Could you check a few things on this model? Use its own coordinates, in mm. Face numbers are marked on the shaded views. A direction names the side the tool comes from. Give positions to 0.01 mm unless a question says otherwise; leave off trailing zeros. Write each loop counter-clockwise with the first axis right and the second up, starting at its lowest first coordinate (ties: lowest second). Pieces come first, ordered by that corner, then holes. Notation, with made-up numbers: M 88,73 L 138,73 A24 ccw 138,98 Z; hole C 38.25,48 d2. An arc over 180 degrees is marked long. One line per item, written item: value.
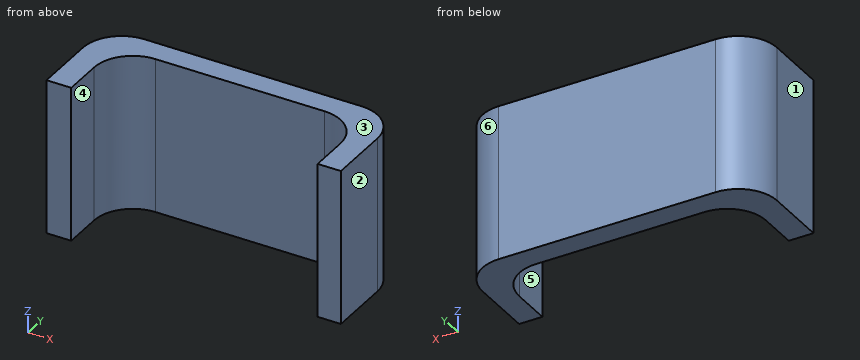
```python
from build123d import *

# Parameters (mm, degrees)
EXTRUDE_1_DEPTH = 40


with BuildPart() as part:
    # 草图1 → 凸台-拉伸1 (new body)
    with BuildSketch(Plane.XY):
        with BuildLine():
            Line((-37.999999813, 14.005326892), (-37.999999813, 20.009487218))
            Line((-37.999999813, 20.009487218), (-37.999999813, 30))
            ThreePointArc((-37.999999813, 30), (-35.071067625, 37.071067812), (-27.999999813, 40))
            Line((-27.999999813, 40), (28, 40))
            ThreePointArc((28, 40), (35.071067812, 37.071067812), (38, 30))
            Line((38, 30), (38, 20))
            Line((38, 20), (38, 14))
            Line((38, 14), (32, 14))
            Line((32, 14), (32, 24))
            ThreePointArc((32, 24), (29.071067812, 31.071067812), (22, 34))
            Line((22, 34), (-21.616055892, 34))
            ThreePointArc((-21.616055892, 34), (-28.687123704, 31.071067812), (-31.616055892, 24))
            Line((-31.616055892, 24), (-31.616055892, 14.005326892))
            Line((-31.616055892, 14.005326892), (-37.999999813, 14.005326892))
        make_face()
    extrude(amount=EXTRUDE_1_DEPTH)


solid = part.part
```
1) I'm going to push flat-ended pins straight in: pin 1 (10 mm diameter, centred on y = 33.5, z = 13.5, fed in from +X); pin 2 (8 mm diameter, centred on x = -10.5, z = 4, fed in from -Y); pin 3 (3 mm diameter, centred on x = -33.5, z = 26.5, fed in from -Y). Where does each tip first touch, or does it pass through?
Outcome:
pin 1: stops at x = 38
pin 2: stops at y = 34
pin 3: stops at y = 14.01
2) If we section it at D-D, the plane y = 26.5: Write out the boundary of the cut face in (x, z).
Outcome:
outline: M -38,0 L -31.3,0 L -31.3,40 L -38,40 Z; M 31.68,0 L 38,0 L 38,40 L 31.68,40 Z
3) We'd pull the mould along X, two halves only. Please class the marked faces 1, 2, 3 and 4: pulls with the +X half, pulls with the -X half, needs draft (parallel to the pull), parting line crosses it, or undercut.
Outcome:
face 1: pulls with the -X half
face 2: pulls with the +X half
face 3: needs draft
face 4: undercut
4) If we section it at A-A, the plane y = 21.25: Write out the boundary of the cut face in (x, z).
Outcome:
outline: M -38,0 L -31.62,0 L -31.62,40 L -38,40 Z; M 32,0 L 38,0 L 38,40 L 32,40 Z
5) If we section it at C-C, the plane x = 12: Write out the boundary of the cut face in (y, z), then the cut area to 3 significant figures.
Outcome:
outline: M 34,0 L 40,0 L 40,40 L 34,40 Z
area: 240 mm^2
6) On a 3-axis mill with a long thin cutter (end or side, diameter ignored), from which of +Z, -Z, +X, -X, +Y, -Y can I reach the whole of each face in a straight line? I mean the marked faces 5 and 6. Say none if no direction works.
Outcome:
face 5: +Z, -Z, -Y
face 6: +Z, -Z, +X, +Y
7) Please list where these lines run through material, in increasing order: L1, parallel to X at y = 16.75, z = 22.5; L2, parallel to Y at x = 8.5, z = 30; L3, parallel to Y at x = 34, z = 16.5. Write a range as from..to.
Outcome:
L1: x = -38..-31.62, 32..38
L2: y = 34..40
L3: y = 14..38
8) If we section it at B-B, the plane z = 35: Write out the boundary of the cut face in (x, y).
Outcome:
outline: M -38,14.01 L -31.62,14.01 L -31.62,24 A10 cw -21.62,34 L 22,34 A10 cw 32,24 L 32,14 L 38,14 L 38,30 A10 ccw 28,40 L -28,40 A10 ccw -38,30 Z
